from build123d import *

# Parameters (mm, degrees)
EXTRUDE_1_DEPTH              = 2
SKETCH_2_W                   = 11
SKETCH_2_H                   = 2
CUT_EXTRUDE_1_DEPTH          = 16.753033088
SKETCH_3_W                   = 11
SKETCH_3_H                   = 2
CUT_EXTRUDE_2_DEPTH          = 16.753033088
EXTRUDE_2_DEPTH              = 8
SKETCH_5_W                   = 47
SKETCH_5_H                   = 2
EXTRUDE_3_DEPTH              = 2
EXTRUDE_START                = 4.4
EXTRUDE_4_DEPTH              = 4.4
CUT_EXTRUDE_3_DEPTH          = 7
HOLE_WIZARD_3_3_3_3_1_D      = 3.3
HOLE_WIZARD_3_3_3_3_1_DEPTH  = 11.5
HOLE_WIZARD_3_3_3_3_1_TIP    = 0.991420021
HOLE_WIZARD_3_3_3_3_2_D      = 3.3
HOLE_WIZARD_3_3_3_3_2_DEPTH  = 11.5
HOLE_WIZARD_3_3_3_3_2_TIP    = 0.991420021
HOLE_WIZARD_10_0_10_1_D      = 10
HOLE_WIZARD_M5_1_D           = 5.5
HOLE_WIZARD_M5_1_DEPTH       = 14.4
HOLE_WIZARD_M5_1_CBORE_D     = 9.5
HOLE_WIZARD_M5_1_CBORE_DEPTH = 5.5
FILLET_1_R                   = 0.5
FILLET_2_R                   = 1
FILLET_4_R                   = 2


with BuildPart() as part:
    # 草图1 → 凸台-拉伸1 (new body)
    with BuildSketch(Plane(origin=(0, 0, 0), x_dir=(-1, 0, 0), z_dir=(0, 0, -1))):
        with BuildLine():
            Line((12.5, -39.153033088), (23.5, -39.153033088))
            Line((23.5, -39.153033088), (23.5, -20.4))
            ThreePointArc((23.5, -20.4), (31.119286624, 0), (23.5, 20.4))
            Line((23.5, 20.4), (-23.5, 20.4))
            ThreePointArc((-23.5, 20.4), (-31.119286624, 0), (-23.5, -20.4))
            Line((-23.5, -20.4), (-23.5, -39.153033088))
            Line((-23.5, -39.153033088), (-12.5, -39.153033088))
            ThreePointArc((-12.5, -39.153033088), (0, -41.1), (12.5, -39.153033088))
        make_face()
    extrude(amount=-EXTRUDE_1_DEPTH)

    # 草图2 → 切除-拉伸1 (cut)
    with BuildSketch(Plane.XZ.offset(39.153033088)):
        with Locations((-18, 1)):
            Rectangle(SKETCH_2_W, SKETCH_2_H)
    extrude(amount=-CUT_EXTRUDE_1_DEPTH, mode=Mode.SUBTRACT)

    # 草图3 → 切除-拉伸2 (cut)
    with BuildSketch(Plane.XZ.offset(39.153033088)):
        with Locations((18, 1)):
            Rectangle(SKETCH_3_W, SKETCH_3_H)
    extrude(amount=-CUT_EXTRUDE_2_DEPTH, mode=Mode.SUBTRACT)

    # 草图4 → 凸台-拉伸2 (add)
    with BuildSketch(Plane.XY.offset(2)):
        with BuildLine():
            Line((-12.5, -39.153033088), (-12.5, -20.4))
            Line((-12.5, -20.4), (-23.5, -20.4))
            ThreePointArc((-23.5, -20.4), (-31.119286624, 0), (-23.5, 20.4))
            Line((-23.5, 20.4), (23.5, 20.4))
            ThreePointArc((23.5, 20.4), (31.119286624, 0), (23.5, -20.4))
            Line((23.5, -20.4), (12.5, -20.4))
            Line((12.5, -20.4), (12.5, -39.153033088))
            ThreePointArc((12.5, -39.153033088), (0, -41.1), (-12.5, -39.153033088))
        make_face()
    extrude(amount=EXTRUDE_2_DEPTH)

    # 草图5 → 凸台-拉伸3 (add)
    with BuildSketch(Plane(origin=(0, 20.4, 0), x_dir=(-1, 0, 0), z_dir=(0, 1, 0))):
        with Locations((0, 1)):
            Rectangle(SKETCH_5_W, SKETCH_5_H)
    extrude(amount=EXTRUDE_3_DEPTH)

    # 草图6 → 凸台-拉伸4 (add)
    with BuildSketch(Plane(origin=(0, 0, 0), x_dir=(-1, 0, 0), z_dir=(0, 0, -1)).offset(EXTRUDE_START)):
        with BuildLine():
            Line((9.188076101, -34.290366833), (10.637462754, -39.69955146))
            ThreePointArc((10.637462754, -39.69955146), (0, -41.1), (-10.637462754, -39.69955146))
            Line((-10.637462754, -39.69955146), (-9.188076101, -34.290366833))
            ThreePointArc((-9.188076101, -34.290366833), (0, -35.5), (9.188076101, -34.290366833))
        make_face()
    extrude(amount=-EXTRUDE_4_DEPTH)

    # 草图7 → 切除-拉伸3 (cut)
    with BuildSketch(Plane.XY.offset(10)):
        with BuildLine():
            Line((9.5, -36.896612311), (9.5, -23.4))
            Line((9.5, -23.4), (-9.5, -23.4))
            Line((-9.5, -23.4), (-9.5, -36.896612311))
            ThreePointArc((-9.5, -36.896612311), (0, -38.1), (9.5, -36.896612311))
        make_face()
    extrude(amount=-CUT_EXTRUDE_3_DEPTH, mode=Mode.SUBTRACT)

    # Ø3.3 (3.3) 直径孔1
    with Locations(Plane(origin=(0, 20.4, 0), x_dir=(1, 0, 0), z_dir=(0, 1, 0))):
        with Locations((-19.5, -6), (19.5, -6), (0, -6)):
            Hole(HOLE_WIZARD_3_3_3_3_1_D / 2, depth=HOLE_WIZARD_3_3_3_3_1_DEPTH)
            with Locations((0, 0, -(HOLE_WIZARD_3_3_3_3_1_DEPTH + HOLE_WIZARD_3_3_3_3_1_TIP / 2))):  # 118° drill point
                Cone(0, HOLE_WIZARD_3_3_3_3_1_D / 2, HOLE_WIZARD_3_3_3_3_1_TIP, mode=Mode.SUBTRACT)

    # Ø3.3 (3.3) 直径孔2
    with Locations(Plane.XZ.offset(20.4)):
        with Locations((-19.5, -6), (-19.5, 6)):
            Hole(HOLE_WIZARD_3_3_3_3_2_D / 2, depth=HOLE_WIZARD_3_3_3_3_2_DEPTH)
            with Locations((0, 0, -(HOLE_WIZARD_3_3_3_3_2_DEPTH + HOLE_WIZARD_3_3_3_3_2_TIP / 2))):  # 118° drill point
                Cone(0, HOLE_WIZARD_3_3_3_3_2_D / 2, HOLE_WIZARD_3_3_3_3_2_TIP, mode=Mode.SUBTRACT)

    # Ø10.0 (10) 直径孔1 (through all)
    with Locations(Plane(origin=(0, 0, 0), x_dir=(-1, 0, 0), z_dir=(0, 0, -1))):
        with Locations((0, 0)):
            Hole(HOLE_WIZARD_10_0_10_1_D / 2)

    # M5 六角头螺栓的柱形沉头孔1
    with Locations(Plane.XY.offset(10)):
        with Locations((16, 0), (8, -13.856406461), (-8, -13.856406461), (-16, 0), (-8, 13.856406461), (8, 13.856406461)):
            CounterBoreHole(HOLE_WIZARD_M5_1_D / 2, HOLE_WIZARD_M5_1_CBORE_D / 2, HOLE_WIZARD_M5_1_CBORE_DEPTH, depth=HOLE_WIZARD_M5_1_DEPTH)

    # 圆角1
    fillet_1_edges = [part.edges().sort_by_distance(p)[0] for p in [
        (23.5, 20.4, 6),
        (-23.5, 20.4, 6),
        (-23.5, -22.4, 1),
        (23.5, -22.4, 1),
        (23.5, -20.4, 6),
        (-23.5, -20.4, 6),
        (23.5, 22.4, 1),
        (-23.5, 22.4, 1),
        (-9.188076101, -34.290366833, -2.2),
        (9.188076101, -34.290366833, -2.2),
        (10.637462754, -39.69955146, -2.2),
        (-10.637462754, -39.69955146, -2.2),
    ]]
    fillet(fillet_1_edges, radius=FILLET_1_R)

    # 圆角2
    fillet_2_edges = [part.edges().sort_by_distance(p)[0] for p in [
        (12.5, -39.153033088, 5),
        (-12.5, -39.153033088, 5),
    ]]
    fillet(fillet_2_edges, radius=FILLET_2_R)

    # 圆角4
    fillet_4_edges = [part.edges().sort_by_distance(p)[0] for p in [
        (9.5, -36.896612311, 6.5),
    ]]
    fillet(fillet_4_edges, radius=FILLET_4_R)


solid = part.part
Work out the finished part from the listing and answer in its coordinate system (mm). A direction names the side the tool comes from. Coordinates: 2 decimals unless noted, no trailing zeros. Loops run counter-clockwise (first coordinate to the right, second up) from the corner with the lowest first, then second, coordinate; pieces in that order, holes last. Notation, with made-up numbers: M 86.25,3 L 124.25,3 A18 cw 124.25,7 Z; hole C 46,-11 d10. An arc over 180 degrees is marked long. Answer in a Markdown table with one row per item. Add a question column.
1. The mould has two halves that part along Z. Classify faces 1 (the flat face through (-9.904, -36.961, -2.231)), 2 (the flat face through (7, -2, 0)), 3 (the cylindrical face through (20.81, 14.57, 7)): pulls with the +Z half, pulls with the -Z half, needs draft (parallel to the pull), parting line crosses it, or undercut.
2. A tool of negligible diameter and unlimited length cuts with its end or side. For faces 4 (the flat face through (-18, -22.4, 1)), 5 (the cylindrical face through (0.4, 14.6, 7.6)), 6 (the cylindrical face through (-18.19, -14.57, 5)), 7 (the cylindrical face through (9.04, -36.59, 6.45)), from which of +Z, -Z, +X, -X, +Y, -Y can it reach the whole face along a straight path? Write none if from no direction.
3. Find section D-D, the plane y = -33.5. Write down the section's boundary in (x, z).
4. Find section C-C, the plane z = -2.5. Write down the section's boundary in (x, y).
5. Find section B-B, the plane y = -2. Write down the section's boundary in (x, z).
6. Flat-ended cylindrical pins translate along their axes: P1, Ø4, axis at x = -22.5, z = 8.5, coming from the -Y side; P2, Ø15, axis at x = 16, y = 0, coming from the -Z side; P3, Ø1.6, axis at x = -18, z = 1, coming from the -Y side. Find the tip coordinate at first contact, or state that the pin passes through.
7. Find section A-A, the plane x = -16. Write down the section's boundary in (y, z).
8. Consider L1, parallel to X at y = -31.5, z = 4.75; L2, parallel to Y at x = -16, z = 6.7; L3, parallel to X at y = 9, z = 6.25. Determine where each line is inside the solid, lowest interval first.
Reported:
| question | item | result |
|---|---|---|
| 1 | face 1 | needs draft |
| 1 | face 2 | pulls with the -Z half |
| 1 | face 3 | undercut |
| 2 | face 4 | +Z, -Z, -X, -Y |
| 2 | face 5 | +Y |
| 2 | face 6 | -Y |
| 2 | face 7 | +Z |
| 3 | outline | M -12.5,0 L 12.5,0 L 12.5,10 L 9.5,10 L 9.5,3 L -9.5,3 L -9.5,10 L -12.5,10 Z |
| 4 | outline | M -10.51,-39.21 A0.5 ccw -10.15,-39.83 A41.1 ccw 10.15,-39.83 A0.5 ccw 10.51,-39.21 L 9.32,-34.77 A0.5 ccw 8.71,-34.41 A35.5 cw -8.71,-34.41 A0.5 ccw -9.32,-34.77 Z |
| 5 | outline | M -31.05,0 L -17.89,0 L -17.89,4.5 L -20.31,4.5 L -20.31,10 L -31.05,10 Z; M -14.11,0 L -4.58,0 L -4.58,10 L -11.69,10 L -11.69,4.5 L -14.11,4.5 Z; M 4.58,0 L 14.11,0 L 14.11,4.5 L 11.69,4.5 L 11.69,10 L 4.58,10 Z; M 17.89,0 L 31.05,0 L 31.05,10 L 20.31,10 L 20.31,4.5 L 17.89,4.5 Z |
| 6 | P1 | stops at y = -20.4 |
| 6 | P2 | stops at z = 0 |
| 6 | P3 | stops at y = -22.4 |
| 7 | outline | M -22.4,0 L -2.75,0 L -2.75,4.5 L -4.75,4.5 L -4.75,10 L -20.4,10 L -20.4,2 L -22.4,2 Z; M 2.75,0 L 22.4,0 L 22.4,2 L 20.4,2 L 20.4,10 L 4.75,10 L 4.75,4.5 L 2.75,4.5 Z |
| 8 | L1 | x = -12.5 to -9.5, 9.5 to 12.5 |
| 8 | L2 | y = -20.4 to -4.75, 4.75 to 20.4 |
| 8 | L3 | x = -29.79 to -21.13, -17.87 to -1.63, 1.63 to 17.87, 21.13 to 29.79 |
